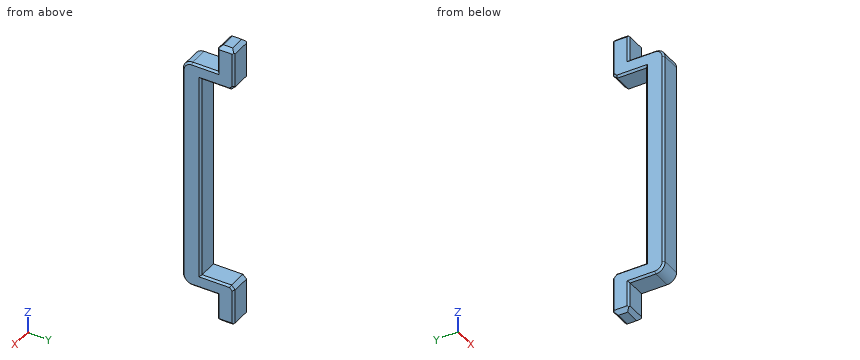
Autodesk Inventor part; units mm, degrees
ref_plane "YZ Plane" through (0, 0, 0) normal (1, 0, 0) x (0, 1, 0)
ref_plane "XZ Plane" through (0, 0, 0) normal (0, 1, 0) x (-1, 0, 0)
ref_plane "XY Plane" through (0, 0, 0) normal (0, 0, 1) x (1, 0, 0)
sketch "スケッチ1" plane through (0, 0, 0) normal (1, 0, 0) x (0, 1, 0)
  line L0 (-6.16, 0) -> (8.96, 0)
  line L1 (0, 43.4) -> (0, -43.4)
  line L2 (0, 22) -> (0, -22)
  line L3 (0, -22) -> (7.1, -22)
  line L4 (7.1, -22) -> (7.1, -31)
  line L5 (7.1, -31) -> (3.5, -31)
  line L6 (3.5, -31) -> (3.5, -25)
  line L7 (3.5, -25) -> (-4, -25)
  line L8 (-4, -25) -> (-4, 25)
  line L9 (-4, 25) -> (3.5, 25)
  line L10 (3.5, 25) -> (3.5, 31)
  line L11 (3.5, 31) -> (7.1, 31)
  line L12 (7.1, 31) -> (7.1, 22)
  line L13 (7.1, 22) -> (0, 22)
  point P0 (0, 0)
  dimension "d0" = 3.5
  dimension "d1" = 4
  dimension "d2" = 50
  dimension "d3" = 6
  dimension "d4" = 3
  dimension "d5" = 3.6
extrude "押し出し1" add sketch "スケッチ1" along normal mid plane 4.8
chamfer "面取り1" distance 0.8 angle 45 10 edges at (0, 7.1, 31) (0, 3.5, 31) (2.4, 5.3, 31) (-2.4, 5.3, 31) (2.4, 5.3, -31) (0, 7.1, -31) (-2.4, 5.3, -31) (0, 3.5, -31) (0, 7.1, 22) (0, 7.1, -22)
fillet "フィレット1" radius 2 2 edges at (0, -4, 25) (0, -4, -25)
chamfer "面取り2" distance 0.4 angle 45 28 edges at (2.4, -4, 0) (2.4, -3.4142, -24.4142) (2.4, 0.75, -25) (2.4, 3.5, -27.6) (2.4, -3.4142, 24.4142) (2.4, 0.75, 25) (2.4, 3.5, 27.6) (-2.4, 0.75, 25) (-2.4, -3.4142, 24.4142) (-2.4, 3.5, 27.6) (-2.4, -4, 0) (-2.4, -3.4142, -24.4142) (-2.4, 0.75, -25) (-2.4, 3.5, -27.6) (2.4, 0, 0) (-2.4, 0, 0) (2.4, 3.15, -22) (2.4, 6.7, -22.4) (2.4, 7.1, -26.5) (-2.4, 7.1, -26.5) (-2.4, 6.7, -22.4) (-2.4, 3.15, -22) (-2.4, 3.15, 22) (-2.4, 6.7, 22.4) (-2.4, 7.1, 26.5) (2.4, 7.1, 26.5) (2.4, 6.7, 22.4) (2.4, 3.15, 22)
properties part number "TrussCC_S1"
CAD build for the part. Positions are in the model's coordinates, mm. Round coordinates to 2 decimals unless told otherwise and drop trailing zeros. Loops run counter-clockwise (first coordinate to the right, second up) from the corner with the lowest first, then second, coordinate; pieces in that order, holes last.
(1) Drop flat-ended pins along their axis: pin 1 (1.2 mm diameter, centred on x = 0.5, y = 2.5, fed in from +Z); pin 2 (1 mm diameter, centred on x = 0.5, y = 2.5, fed in from -Z); pin 3 (2 mm diameter, centred on x = -0.5, z = 27.5, fed in from -Y); pin 4 (6 mm diameter, centred on y = 4, z = -14, fed in from +X). Give the stop position or say it passes through.
(2) Cut at A-A (z = 3). Give the cut face in (x, y), plus the area to 3 significant figures.
(3) Cut at B-B (x = 0.4). Give the cut face in (y, z), plus the area to 3 significant figures.
(4) Wall check: line 1 along Z through (x, y) = (0.8, 2.25); line 2 along Y through (x, z) = (-1.1, 2.5); line 3 along Z through (x, y) = (2, -2). Give the ranges that are in metal, low to high.
Findings below:
1. pin 1: stops at z = 25
1. pin 2: stops at z = -25
1. pin 3: stops at y = 3.5
1. pin 4: passes through
2. outline: (-2.4, -3.6) - (-2, -4) - (2, -4) - (2.4, -3.6) - (2.4, -0.4) - (2, 0) - (-2, 0) - (-2.4, -0.4) - close
2. area: 18.9 mm2
3. outline: (-4, -23) arc R2 ccw to (-2, -25) - (3.5, -25) - (3.5, -30.2) - (4.3, -31) - (6.3, -31) - (7.1, -30.2) - (7.1, -22.8) - (6.3, -22) - (0, -22) - (0, 22) - (6.3, 22) - (7.1, 22.8) - (7.1, 30.2) - (6.3, 31) - (4.3, 31) - (3.5, 30.2) - (3.5, 25) - (-2, 25) arc R2 ccw to (-4, 23) - close
3. area: 282 mm2
4. line 1: z = -25 to -22, 22 to 25
4. line 2: y = -4 to 0
4. line 3: z = -25 to 25
